```python
from build123d import *

# Parameters (mm, degrees)
SKETCH_1_W                   = 40
SKETCH_1_H                   = 40
EXTRUDE_1_DEPTH              = 1.5
SKETCH_2_R                   = 1.75
CUT_EXTRUDE_1_DEPTH          = 29.324018077
EXTRUDE_START                = -1.5
SKETCH_3_W                   = 1.5
SKETCH_3_H                   = 40
EXTRUDE_2_DEPTH              = 47
SKETCH_4_R                   = 1.5
CUT_EXTRUDE_2_DEPTH          = 65.876806333
HOLE_WIZARD_M3_1_D           = 3.4
HOLE_WIZARD_M3_1_DEPTH       = 15
HOLE_WIZARD_M3_1_CSINK_D     = 7.1
HOLE_WIZARD_M3_1_CSINK_ANGLE = 92
HOLE_WIZARD_M3_1_TIP         = 1.021463052
FILLET_1_R                   = 20
FILLET_2_R                   = 1


with BuildPart() as part:
    # 스케치1 → 보스-돌출1 (new body)
    with BuildSketch(Plane(origin=(0, 0, 0), x_dir=(1, 0, 0), z_dir=(0, 1, 0))):
        Rectangle(SKETCH_1_W, SKETCH_1_H)
    extrude(amount=EXTRUDE_1_DEPTH)

    # 스케치2 → 컷-돌출1 (cut, through all)
    with BuildSketch(Plane(origin=(0, 1.5, 0), x_dir=(1, 0, 0), z_dir=(0, 1, 0))):
        with Locations(Location((-12, 15, 0), (0, 0, 270))):
            Circle(SKETCH_2_R)
        with Locations(Location((12, 15, 0), (0, 0, 270))):
            Circle(SKETCH_2_R)
        with Locations(Location((-12, -15, 0), (0, 0, 270))):
            Circle(SKETCH_2_R)
        with Locations(Location((12, -15, 0), (0, 0, 270))):
            Circle(SKETCH_2_R)
    extrude(amount=-CUT_EXTRUDE_1_DEPTH, mode=Mode.SUBTRACT)

    # 스케치3 → 보스-돌출2 (add)
    with BuildSketch(Plane(origin=(0, 1.5, 0), x_dir=(1, 0, 0), z_dir=(0, 1, 0)).offset(EXTRUDE_START)):
        with Locations((19.25, 0)):
            Rectangle(SKETCH_3_W, SKETCH_3_H)
    extrude(amount=EXTRUDE_2_DEPTH)

    # 스케치4 → 컷-돌출2 (cut, through all)
    with BuildSketch(Plane(origin=(20, 0, 0), x_dir=(0, 0, -1), z_dir=(1, 0, 0))):
        with Locations((15.5, 27)):
            Circle(SKETCH_4_R)
        with Locations((7.75, 13.576606241)):
            Circle(SKETCH_4_R)
        with Locations((-7.75, 13.576606241)):
            Circle(SKETCH_4_R)
        with Locations((-15.5, 27)):
            Circle(SKETCH_4_R)
        with Locations((-7.75, 40.423393759)):
            Circle(SKETCH_4_R)
        with Locations((7.75, 40.423393759)):
            Circle(SKETCH_4_R)
        with BuildLine():
            Line((-6.5, 20), (-6.5, 34))
            ThreePointArc((-6.5, 34), (0, 40.5), (6.5, 34))
            Line((6.5, 34), (6.5, 20))
            ThreePointArc((6.5, 20), (0, 13.5), (-6.5, 20))
        make_face()
    extrude(amount=-CUT_EXTRUDE_2_DEPTH, mode=Mode.SUBTRACT)

    # M3 둥근 십자머리 나사용 카운터싱크1
    with Locations(Plane(origin=(20, 0, 0), x_dir=(0, 0, -1), z_dir=(1, 0, 0))):
        with Locations((15.5, 27), (7.75, 40.423393759), (-7.75, 40.423393759), (-15.5, 27), (-7.75, 13.576606241), (7.75, 13.576606241)):
            CounterSinkHole(HOLE_WIZARD_M3_1_D / 2, HOLE_WIZARD_M3_1_CSINK_D / 2, depth=HOLE_WIZARD_M3_1_DEPTH, counter_sink_angle=HOLE_WIZARD_M3_1_CSINK_ANGLE)
            with Locations((0, 0, -(HOLE_WIZARD_M3_1_DEPTH + HOLE_WIZARD_M3_1_TIP / 2))):  # 118° drill point
                Cone(0, HOLE_WIZARD_M3_1_D / 2, HOLE_WIZARD_M3_1_TIP, mode=Mode.SUBTRACT)

    # 필렛1
    fillet_1_edges = [part.edges().sort_by_distance(p)[0] for p in [
        (19.25, 47, -20),
        (19.25, 47, 20),
    ]]
    fillet(fillet_1_edges, radius=FILLET_1_R - 0.0001)  # a hair under: the kernel refuses the full size

    # 필렛2
    fillet_2_edges = [part.edges().sort_by_distance(p)[0] for p in [
        (18.5, 1.5, 0),
        (20, 0, 0),
        (-20, 0.75, 20),
        (-20, 0.75, -20),
    ]]
    fillet(fillet_2_edges, radius=FILLET_2_R)


solid = part.part
```
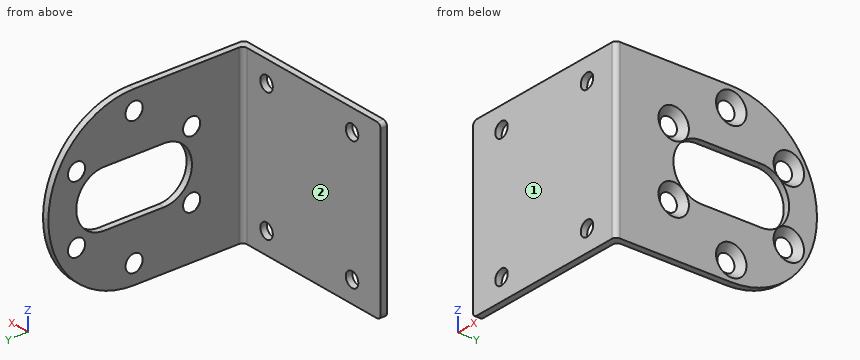
Geometry check sheet. Reference: the model listing, model coordinates, mm. Face numbers are marked on the shaded views. A direction names the side the tool comes from. Give positions to 0.01 mm unless a question says otherwise; leave off trailing zeros. Order: outer loops, then holes, each group sorted by start corner. A loop starts at its lowest first (then second) coordinate and runs counter-clockwise, first axis right, second up.
1. Section check D-D, the plane y = 36. Enter the section's corners in (x, z), and give its area (3 significant figures).
2. Section check A-A, the plane y = 22. Enter the section's corners in (x, z).
3. Access from +Z, -Z, +X, -X, +Y, -Y to the whole of each face (thin tool, end or side, straight path). Record for the marked faces 1 and 2.
4. Section check B-B, the plane x = 12. Enter the section's corners in (y, z), and give its area (3 significant figures).
5. Thickness scan on L1, parallel to X at y = 1, z = -15; L2, parallel to Y at x = -13, z = 13.5; L3, parallel to X at y = 20.5, z = -11.5. Record the ranges inside material, lowest first.
6. Gauge pin test, flat ends, axial feed: pin 1 Ø5.5 at (x, z) = (-12, -15) entering from +Y; pin 2 Ø1.6 at (x, y) = (19.5, 29) entering from -Z; pin 3 Ø0.8 at (x, y) = (19.5, 30) entering from +Z; pin 4 Ø3 at (x, z) = (12, -15) entering from -Y. Record the tip position at first contact, or that the pin passes through.
7. Section check C-C, the plane z = 15.5. Enter the section's corners in (x, y), and give its area (3 significant figures).
Values follow:
1. outline: (18.5, -17.86) - (20, -17.86) - (20, -6.18) - (18.5, -6.18) - close; (18.5, 6.18) - (20, 6.18) - (20, 17.86) - (18.5, 17.86) - close
1. area: 35.0 mm2
2. outline: (18.5, -20) - (20, -20) - (20, -6.5) - (18.5, -6.5) - close; (18.5, 6.5) - (20, 6.5) - (20, 20) - (18.5, 20) - close
3. face 1: +Z, -Z, +X, -X, -Y
3. face 2: +Z, -Z, -X, +Y
4. outline: (0, -20) - (1.5, -20) - (1.5, -16.75) - (0, -16.75) - close; (0, -13.25) - (1.5, -13.25) - (1.5, 13.25) - (0, 13.25) - close; (0, 16.75) - (1.5, 16.75) - (1.5, 20) - (0, 20) - close
4. area: 49.5 mm2
5. L1: x = -20 to -13.75, -10.25 to 10.25, 13.75 to 20
5. L2: y = 0 to 1.5
5. L3: x = 18.5 to 20
6. pin 1: stops at y = 1.5
6. pin 2: stops at z = -19.96
6. pin 3: stops at z = 19.83
6. pin 4: passes through
7. outline: (-20, 0) - (-13.68, 0) - (-13.68, 1.5) - (-20, 1.5) - close; (-10.32, 0) - (10.32, 0) - (10.32, 1.5) - (-10.32, 1.5) - close; (13.68, 0) - (19, 0) arc R1 ccw to (20, 1) - (20, 23.45) - (18.5, 25) - (18.5, 2.5) arc R1 cw to (17.5, 1.5) - (13.68, 1.5) - close; (18.5, 29) - (20, 30.55) - (20, 39.64) - (18.5, 39.64) - close
7. area: 98.8 mm2
